Verification items for the finished model (mm, model axes). Coordinates: 2 decimals unless noted, no trailing zeros. Write each loop counter-clockwise with the first axis right and the second up, starting at its lowest first coordinate (ties: lowest second). Pieces come first, ordered by that corner, then holes. Notation, with made-up numbers: (-3.75, 87.5) -> (39.25, 87.5) arc R16 ccw to (39.25, 103.5) -> close; hole circle Ø3 at (13.25, -11.5). An arc over 180 degrees is marked (long way). Answer in a Markdown table with one row per item.
```python
from build123d import *

# Parameters (mm, degrees)
CROQUIS1_W              = 250
CROQUIS1_H              = 150
SALIENTE_EXTRUIR1_DEPTH = 3
REDONDEO1_R             = 15
CORTAR_EXTRUIR1_REACH   = 147.805
CROQUIS2_R              = 2.25
CROQUIS3_R              = 4
CORTAR_EXTRUIR2_DEPTH   = 5
CROQUIS4_R              = 11
CROQUIS4_R_2            = 8.15
SALIENTE_EXTRUIR2_DEPTH = 6
REDONDEO2_R             = 2
CROQUIS5_R              = 25
CROQUIS5_R_2            = 20
SALIENTE_EXTRUIR3_DEPTH = 20
REDONDEO3_R             = 20
REDONDEO4_R             = 5
CROQUIS11_W             = 60
CROQUIS11_H             = 8
CORTAR_EXTRUIR6_DEPTH   = 20
REDONDEO7_R             = 1
CROQUIS12_R             = 10
CORTAR_EXTRUIR7_DEPTH   = 200
CROQUIS6_R              = 2
CORTAR_EXTRUIR8_DEPTH   = 10


with BuildPart() as part:
    # Croquis1 → Saliente-Extruir1 (new body)
    with BuildSketch(Plane(origin=(0, 0, 0), x_dir=(1, 0, 0), z_dir=(0, 1, 0))):
        Rectangle(CROQUIS1_W, CROQUIS1_H)
    extrude(amount=SALIENTE_EXTRUIR1_DEPTH)

    # Redondeo1
    redondeo1_edges = [part.edges().sort_by_distance(p)[0] for p in [
        (125, 1.5, 75),
        (-125, 1.5, 75),
        (-125, 1.5, -75),
        (125, 1.5, -75),
    ]]
    fillet(redondeo1_edges, radius=REDONDEO1_R)

    # Croquis2 → Cortar-Extruir1 (cut, up to next)
    with BuildSketch(Plane(origin=(0, 3, 0), x_dir=(1, 0, 0), z_dir=(0, 1, 0)), mode=Mode.PRIVATE) as cortar_extruir1_sk1:
        with Locations(Location((-115, 65, 0), (0, 0, 270))):
            Circle(CROQUIS2_R)
    cortar_extruir1_tool1 = extrude(cortar_extruir1_sk1.sketch, amount=-CORTAR_EXTRUIR1_REACH, mode=Mode.PRIVATE) & part.part
    # Croquis2 → Cortar-Extruir1 (cut, up to next)
    with BuildSketch(Plane(origin=(0, 3, 0), x_dir=(1, 0, 0), z_dir=(0, 1, 0)), mode=Mode.PRIVATE) as cortar_extruir1_sk2:
        with Locations(Location((115, 65, 0), (0, 0, 270))):
            Circle(CROQUIS2_R)
    cortar_extruir1_tool2 = extrude(cortar_extruir1_sk2.sketch, amount=-CORTAR_EXTRUIR1_REACH, mode=Mode.PRIVATE) & part.part
    # Croquis2 → Cortar-Extruir1 (cut, up to next)
    with BuildSketch(Plane(origin=(0, 3, 0), x_dir=(1, 0, 0), z_dir=(0, 1, 0)), mode=Mode.PRIVATE) as cortar_extruir1_sk3:
        with Locations(Location((115, -65, 0), (0, 0, 270))):
            Circle(CROQUIS2_R)
    cortar_extruir1_tool3 = extrude(cortar_extruir1_sk3.sketch, amount=-CORTAR_EXTRUIR1_REACH, mode=Mode.PRIVATE) & part.part
    # Croquis2 → Cortar-Extruir1 (cut, up to next)
    with BuildSketch(Plane(origin=(0, 3, 0), x_dir=(1, 0, 0), z_dir=(0, 1, 0)), mode=Mode.PRIVATE) as cortar_extruir1_sk4:
        with Locations(Location((-115, -65, 0), (0, 0, 270))):
            Circle(CROQUIS2_R)
    cortar_extruir1_tool4 = extrude(cortar_extruir1_sk4.sketch, amount=-CORTAR_EXTRUIR1_REACH, mode=Mode.PRIVATE) & part.part
    add(cortar_extruir1_tool1.solids().sort_by_distance((-115, 3, -65))[0], mode=Mode.SUBTRACT)
    add(cortar_extruir1_tool2.solids().sort_by_distance((115, 3, -65))[0], mode=Mode.SUBTRACT)
    add(cortar_extruir1_tool3.solids().sort_by_distance((115, 3, 65))[0], mode=Mode.SUBTRACT)
    add(cortar_extruir1_tool4.solids().sort_by_distance((-115, 3, 65))[0], mode=Mode.SUBTRACT)

    # Croquis3 → Cortar-Extruir2 (cut)
    with BuildSketch(Plane(origin=(0, 3, 0), x_dir=(1, 0, 0), z_dir=(0, 1, 0))):
        with Locations(Location((-75, 0, 0), (0, 0, 270))):
            Circle(CROQUIS3_R)
    extrude(amount=-CORTAR_EXTRUIR2_DEPTH, mode=Mode.SUBTRACT)

    # Croquis4 → Saliente-Extruir2 (add)
    with BuildSketch(Plane(origin=(0, 3, 0), x_dir=(1, 0, 0), z_dir=(0, 1, 0))):
        with Locations(Location((-75, 0, 0), (0, 0, 90))):
            Circle(CROQUIS4_R)
        with Locations(Location((-75, 0, 0), (0, 0, 270))):
            Circle(CROQUIS4_R_2, mode=Mode.SUBTRACT)
    extrude(amount=SALIENTE_EXTRUIR2_DEPTH)

    # Redondeo2
    redondeo2_edges = [part.edges().sort_by_distance(p)[0] for p in [
        (-75, 3, 11),
    ]]
    fillet(redondeo2_edges, radius=REDONDEO2_R)

    # Croquis5 → Saliente-Extruir3 (add)
    with BuildSketch(Plane(origin=(0, 3, 0), x_dir=(1, 0, 0), z_dir=(0, 1, 0))):
        with Locations(Location((95, 35, 0), (0, 0, 90))):
            Circle(CROQUIS5_R)
        with Locations(Location((95, 35, 0), (0, 0, 270))):
            Circle(CROQUIS5_R_2, mode=Mode.SUBTRACT)
    extrude(amount=SALIENTE_EXTRUIR3_DEPTH)

    # Redondeo3
    redondeo3_edges = [part.edges().sort_by_distance(p)[0] for p in [
        (95, 3, -55),
    ]]
    fillet(redondeo3_edges, radius=REDONDEO3_R - 0.0001)  # a hair under: the kernel refuses the full size

    # Redondeo4
    redondeo4_edges = [part.edges().sort_by_distance(p)[0] for p in [
        (95, 3, -10),
    ]]
    fillet(redondeo4_edges, radius=REDONDEO4_R - 0.0001)  # a hair under: the kernel refuses the full size

    # Croquis11 → Cortar-Extruir6 (cut)
    with BuildSketch(Plane(origin=(0, 3, 0), x_dir=(1, 0, 0), z_dir=(0, 1, 0))):
        with Locations((35, 46)):
            Rectangle(CROQUIS11_W, CROQUIS11_H)
    extrude(amount=-CORTAR_EXTRUIR6_DEPTH, mode=Mode.SUBTRACT)

    # Redondeo7
    redondeo7_edges = [part.edges().sort_by_distance(p)[0] for p in [
        (5, 1.5, -42),
        (5, 1.5, -50),
        (65, 1.5, -50),
        (65, 1.5, -42),
    ]]
    fillet(redondeo7_edges, radius=REDONDEO7_R)

    # Croquis12 → Cortar-Extruir7 (cut)
    with BuildSketch(Plane(origin=(0, 3, 0), x_dir=(1, 0, 0), z_dir=(0, 1, 0))):
        with Locations(Location((30.572379794, -49.649260846, 0), (0, 0, 270))):
            Circle(CROQUIS12_R)
    extrude(amount=-CORTAR_EXTRUIR7_DEPTH, mode=Mode.SUBTRACT)

    # Croquis6 → Cortar-Extruir8 (cut)
    with BuildSketch(Plane(origin=(0, 3, 0), x_dir=(1, 0, 0), z_dir=(0, 1, 0))):
        with Locations(Location((113.5, -1.5, 0), (0, 0, 270))):
            Circle(CROQUIS6_R)
        with Locations(Location((113.5, -38.5, 0), (0, 0, 270))):
            Circle(CROQUIS6_R)
        with Locations(Location((76.5, -38.5, 0), (0, 0, 270))):
            Circle(CROQUIS6_R)
        with Locations(Location((76.5, -1.5, 0), (0, 0, 270))):
            Circle(CROQUIS6_R)
    extrude(amount=-CORTAR_EXTRUIR8_DEPTH, mode=Mode.SUBTRACT)


solid = part.part
```
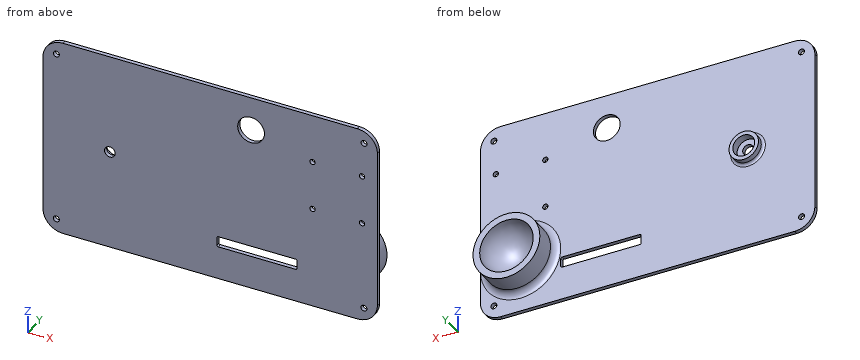
1. Go/stop test with flat-tipped pins: pin 1 (3.5 mm diameter, centred on x = 115, z = 65, fed in from +Y); pin 2 (8 mm diameter, centred on y = 11.5, z = -58.5, fed in from -X); pin 3 (24 mm diameter, centred on x = -75, z = 4.5, fed in from +Y); pin 4 (2 mm diameter, centred on y = 13.5, z = -15, fed in from +X). Record where each tip stops, or that it passes through.
Findings below:
| item | result |
|---|---|
| pin 1 | passes through |
| pin 2 | stops at x = 79.36 |
| pin 3 | stops at y = 9 |
| pin 4 | stops at x = 111.25 |
2. Sectioned sample at A-A, the plane x = 61. Record the cut outline in (y, z), and give its area (3 significant figures).
Findings below:
| item | result |
|---|---|
| outline | (0, -75) -> (3, -75) -> (3, -50) -> (0, -50) -> close; (0, -42) -> (3, -42) -> (3, 75) -> (0, 75) -> close |
| area | 426 mm² |
3. Sectioned sample at B-B, the plane x = -75. Record the cut outline in (y, z).
Findings below:
| item | result |
|---|---|
| outline | (0, -75) -> (3, -75) -> (3, -13) arc R2 cw to (5, -11) -> (9, -11) -> (9, -8.15) -> (3, -8.15) -> (3, -4) -> (0, -4) -> close; (0, 4) -> (3, 4) -> (3, 8.15) -> (9, 8.15) -> (9, 11) -> (5, 11) arc R2 cw to (3, 13) -> (3, 75) -> (0, 75) -> close |
4. Sectioned sample at D-D, the plane x = -100. Record the cut outline in (y, z).
Findings below:
| item | result |
|---|---|
| outline | (0, -75) -> (3, -75) -> (3, 75) -> (0, 75) -> close |
5. Sectioned sample at C-C, the plane z = 33. Record the cut outline in (x, y).
Findings below:
| item | result |
|---|---|
| outline | (-125, 0) -> (125, 0) -> (125, 3) -> (-125, 3) -> close |
6. Material ranges on probe 1 along X at (y, z) = (1.4, 38.5); probe 2 along X at (y, z) = (1.95, -65); probe 3 along X at (y, z) = (1.45, 1.5), recorded low to high. Write a range as from..to.
Findings below:
| item | result |
|---|---|
| probe 1 | x = -125..74.5, 78.5..111.5, 115.5..125 |
| probe 2 | x = -124.14..-117.25, -112.75..112.75, 117.25..124.14 |
| probe 3 | x = -125..-78.71, -71.29..74.5, 78.5..111.5, 115.5..125 |
